```python
from build123d import *

# Parameters (mm, degrees)
BOSS_EXTRUDE1_DEPTH = 60
SKETCH2_R           = 2.5
CUT_EXTRUDE1_DEPTH  = 106.148276258


with BuildPart() as part:
    # Sketch1 → Boss-Extrude1 (new body)
    with BuildSketch(Plane(origin=(0, 0, 0), x_dir=(1, 0, 0), z_dir=(0, 1, 0))):
        Polygon((0, 0), (0, 70.4), (3, 70.4), (3, 3), (50, 3), (50, 0), align=None)
    extrude(amount=BOSS_EXTRUDE1_DEPTH)

    # Sketch2 → Cut-Extrude1 (cut, through all)
    with BuildSketch(Plane.ZY):
        with Locations((-63.4, 6)):
            Circle(SKETCH2_R)
        with Locations((-15.4, 6)):
            Circle(SKETCH2_R)
        with Locations((-15.4, 54)):
            Circle(SKETCH2_R)
        with Locations((-63.4, 54)):
            Circle(SKETCH2_R)
    extrude(amount=-CUT_EXTRUDE1_DEPTH, mode=Mode.SUBTRACT)


solid = part.part
```
Geometry: final body of the model. Coordinates: model frame, mm. A direction names the side the tool comes from. Coordinates: 2 decimals unless noted, no trailing zeros. Order: outer loops, then holes, each group sorted by start corner. A loop starts at its lowest first (then second) coordinate and runs counter-clockwise, first axis right, second up. Notation, with made-up numbers: (33.25, 16.5) -> (79.25, 16.5) arc R13 cw to (79.25, 20.5) -> close; hole circle Ø3 at (9, 53.5). An arc over 180 degrees is marked (long way). Write item = value, one per line.
(1) Pull-direction query (Y, two-part tool) for faces 1 (the flat face through (1, 0, -25)), 2 (the cylindrical face through (1.48, 53.04, -61.09)), 3 (the flat face through (50, 30, -2)); classes: pulls with the +Y half, pulls with the -Y half, needs draft (parallel to the pull), parting line crosses it, or undercut.
Solved:
face_1 = pulls with the -Y half
face_2 = undercut
face_3 = needs draft
(2) Pin query (flat end, axial travel): pin 1 Ø4 at (y, z) = (6, -63.4) entering from +X; pin 2 Ø4 at (x, y) = (16.5, 45) entering from -Z; pin 3 Ø1.5 at (y, z) = (8.5, -45) entering from +X. Return the tip coordinate at first contact, or that it passes through.
Solved:
pin_1 = through
pin_2 = -3
pin_3 = 3
(3) Cut plane A-A on y = 6. Return loops of the section in (x, z).
Solved:
outline = (0, -70.4) -> (3, -70.4) -> (3, -65.9) -> (0, -65.9) -> close; (0, -60.9) -> (3, -60.9) -> (3, -17.9) -> (0, -17.9) -> close; (0, -12.9) -> (3, -12.9) -> (3, -3) -> (50, -3) -> (50, 0) -> (0, 0) -> close
(4) Cut plane C-C on y = 41. Return loops of the section in (x, z), plus the area to 3 significant figures.
Solved:
outline = (0, -70.4) -> (3, -70.4) -> (3, -3) -> (50, -3) -> (50, 0) -> (0, 0) -> close
area = 352 mm²
(5) Cut plane B-B on z = -63.4. Return loops of the section in (x, y).
Solved:
outline = (0, 0) -> (3, 0) -> (3, 3.5) -> (0, 3.5) -> close; (0, 8.5) -> (3, 8.5) -> (3, 51.5) -> (0, 51.5) -> close; (0, 56.5) -> (3, 56.5) -> (3, 60) -> (0, 60) -> close
(6) Line query: line 1 (Y direction, x = 2.15, z = -15.4); line 2 (Z direction, x = 48.5, y = 27.5); line 3 (X direction, y = 43, z = -30.5). Output: solid intervals per line, ascending.
Solved:
line_1 = 0 to 3.5, 8.5 to 51.5, 56.5 to 60
line_2 = -3 to 0
line_3 = 0 to 3
(7) Access query for faces 4 (the flat face through (26, 30, -3)), 5 (the cylindrical face through (1.5, 6.1, -17.9)). Directions: +Z, -Z, +X, -X, +Y, -Y. A direction counts if a zero-diameter tool reaches every point of the face in a straight line with its end or side. Return the directions, or none.
Solved:
face_4 = -Z, +X, +Y, -Y
face_5 = +X, -X
(8) Cut plane D-D on x = 40. Return loops of the section in (y, z).
Solved:
outline = (0, -3) -> (60, -3) -> (60, 0) -> (0, 0) -> close
